The model under review builds one solid part; all positions refer to its coordinate system, in mm. Give positions to 0.01 mm unless a question says otherwise; leave off trailing zeros. Order: outer loops, then holes, each group sorted by start corner. A loop starts at its lowest first (then second) coordinate and runs counter-clockwise, first axis right, second up.
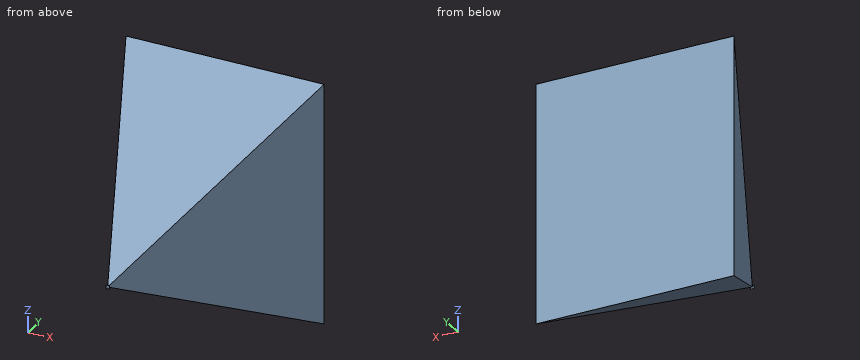
Autodesk Inventor part; units mm, degrees
ref_plane "YZ Plane" through (0, 0, 0) normal (1, 0, 0) x (0, 1, 0)
ref_plane "XZ Plane" through (0, 0, 0) normal (0, 1, 0) x (-1, 0, 0)
ref_plane "XY Plane" through (0, 0, 0) normal (0, 0, 1) x (1, 0, 0)
sketch "Sketch1" plane through (0, 0, 0) normal (0, 1, 0) x (-1, 0, 0)
  line L0 (0, 0) -> (550, 0)
  line L1 (550, 0) -> (550, -670)
  line L2 (550, -670) -> (0, -670)
  line L3 (0, -670) -> (0, 0)
  dimension "d0" = 670
  dimension "d1" = 550
extrude "Extrusion1" add sketch "Sketch1" along normal blind 630
sketch "Sketch5" plane through (0, 0, 0) normal (1, 0, 0) x (0, 0, -1)
  line L0 (0, 630) -> (0, 0)
  line L1 (0, 0) -> (335, 0)
  line L2 (0, 0) -> (670, 0)
  line L3 (0, 630) -> (335, 0)
extrude "Extrusion2" cut sketch "Sketch5" against normal through all
sketch "Sketch6" plane through (0, 0, -670) normal (1, 0, 0) x (0, 0, -1)
  line L0 (-670, 630) -> (-335, 0)
  line L1 (-335, 0) -> (0, 630)
  line L2 (0, 630) -> (0, 0)
  line L3 (0, 0) -> (-335, 0)
  point P0 (-670, 0)
extrude "Extrusion3" cut sketch "Sketch6" against normal through all
sketch "Sketch8" plane through (0, 0, 0) normal (0, 0, 1) x (1, 0, 0)
  line L0 (-550, 630) -> (0, 630)
  line L1 (-550, 0) -> (-550, 630)
  line L2 (-550, 630) -> (-550, 0)
  line L3 (-550, 0) -> (-275, 0)
  line L4 (-275, 0) -> (-550, 630)
  point P0 (0, 0)
  dimension "d8" = 275
extrude "Extrusion4" cut sketch "Sketch8" against normal through all
sketch "Sketch9" plane through (0, 0, 0) normal (0, 0, 1) x (1, 0, 0)
  line L0 (0, 0) -> (-275, 0)
  line L1 (-275, 0) -> (0, 630)
  line L2 (0, 630) -> (0, 0)
extrude "Extrusion5" cut sketch "Sketch9" against normal through all
sketch "Sketch10" plane through (0, 0, 0) normal (0, 1, 0) x (-1, 0, 0)
  line L0 (270, -330) -> (280, -330)
  line L1 (280, -330) -> (280, -340)
  line L2 (280, -340) -> (270, -340)
  line L3 (270, -340) -> (270, -330)
  line L4 (550, 0) -> (0, 0)
  line L5 (0, 0) -> (0, -670)
  dimension "d13" = 10
  dimension "d14" = 10
  dimension "d15" = 330
  dimension "d16" = 270
extrude "Extrusion6" add sketch "Sketch10" along normal blind 0.1
properties part number "FieldofView"
Item 1: Clearance check with flat-ended pins moving along their axes: pin 1 Ø8 at (x, y) = (-170.5, 539.5) entering from -Z; pin 2 Ø2 at (x, y) = (-474, 499) entering from +Z; pin 3 Ø12 at (x, z) = (-435.5, -434) entering from -Y. State where each tip first meets the part, or that it passes through.
Values found:
pin 1: stops at z = -624
pin 2: stops at z = -69.13
pin 3: stops at y = 353.95
Item 2: Take a section at B-B (z = -427). Give the boundary of the cut face in (x, y).
Values found:
outline: (-550, 630) - (-350.52, 173.01) - (-199.48, 173.01) - (0, 630) - close
Item 3: Take a section at A-A (x = -242). Give the boundary of the cut face in (y, z), and give its area (3 significant figures).
Values found:
outline: (75.6, -375.2) - (630, -670) - (630, 0) - (75.6, -294.8) - close
area: 208,000 mm2
Item 4: For line 1 (Z direction, x = -74, y = 542); line 2 (Z direction, x = -458.5, y = 553.5); line 3 (Y direction, x = -324, z = -419), list the stretches that pass through material, from the lowest coordinate up.
Values found:
line 1: z = -623.21 to -46.79
line 2: z = -629.32 to -40.68
line 3: y = 157.97 to 630
